Read the model definition and answer for the solid it produces. Units are mm, in the model's axes. Round coordinates to 2 decimals unless told otherwise and drop trailing zeros. Order: outer loops, then holes, each group sorted by start corner. A loop starts at its lowest first (then second) coordinate and runs counter-clockwise, first axis right, second up. Notation, with made-up numbers: (51.5, 25) - (92.5, 25) arc R28 ccw to (92.5, 45) - close; hole circle Ø9 at (86, 22.5). An arc over 180 degrees is marked (long way). Put each result on its own line as item: value. Start each with the question number.
Q1. Section B-B on y = -107.5 is taken. Give the vertices of the cut face in (x, z), then the cut area to 3 significant figures.
Q2. Section C-C on z = 100 is taken. Give the vertices of the cut face in (x, y), then the cut area to 3 significant figures.
Q3. Section A-A on z = -730.5 is taken. Give the vertices of the cut face in (x, y), then the cut area to 3 significant figures.
Q4. Each of these flat-tipped pins is pushed along its axis until it touches: pin 1 Ø5 at (x, y) = (422.5, -30.5) entering from +Z; pin 2 Ø3 at (y, z) = (-62, 583.5) entering from +X; pin 3 Ø1.5 at (x, y) = (-468, -133) entering from +Z. Where does it stop, or does it pass through?
Q5. Section D-D on x = 264 is taken. Give the vertices of the cut face in (y, z), then the cut area to 3 significant figures.
Q6. Find the intervals of material crossed by line 1 along X through (y, z) = (-67, -637); line 2 along Z through (x, y) = (-70.5, -88.5); line 3 along X through (y, z) = (-120.5, 274), in increasing order. Write a range as from..to.
from build123d import *

# Parameters (mm, degrees)
F1_DEPTH = 152.4
F2_W     = 1219.2
F2_H     = 1828.8
F3_DEPTH = 25.4
F4_DEPTH = 152.401


with BuildPart() as f1:
    # F0 (on Front) → F1 (new body)
    with BuildSketch(Plane.XZ):
        with BuildLine():
            Line((-962.472789, 62.231022), (-962.472789, -1309.368978))
            Line((-962.472789, -1309.368978), (866.327211, -1309.368978))
            Line((866.327211, -1309.368978), (866.327211, 62.231022))
            ThreePointArc((866.327211, 62.231022), (-48.072789, 976.631022), (-962.472789, 62.231022))
        make_face()
    extrude(amount=F1_DEPTH)

    # F2 (on face) → F3 (cut)
    with BuildSketch(Plane.XZ.offset(152.4)):
        with Locations((-48.072789, -394.968978)):
            Rectangle(F2_W, F2_H)
    extrude(amount=-F3_DEPTH, mode=Mode.SUBTRACT)

    # F2 (on face) → F4 (cut, through all)
    with BuildSketch(Plane.XZ.offset(152.4)):
        with Locations((-48.072789, -394.968978)):
            Rectangle(F2_W, F2_H)
    extrude(amount=-F4_DEPTH, mode=Mode.SUBTRACT)


solid = f1.part
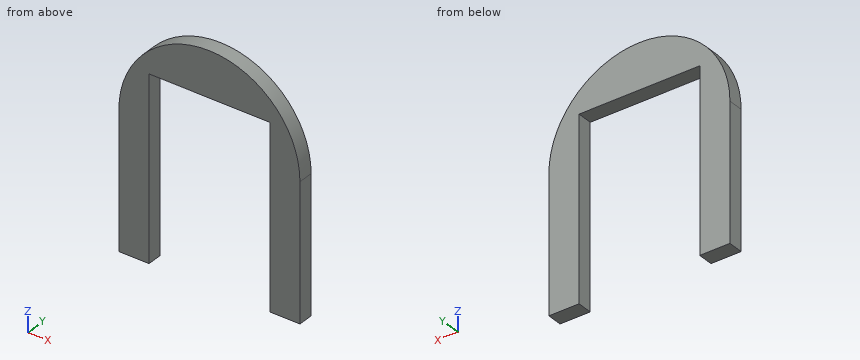
Findings:
1. outline: (-962.47, -1309.37) - (-657.67, -1309.37) - (-657.67, 519.43) - (561.53, 519.43) - (561.53, -1309.37) - (866.33, -1309.37) - (866.33, 62.23) arc R914.4 ccw to (-962.47, 62.23) - close
1. area: 1,590,000 mm2
2. outline: (-961.69, -152.4) - (-657.67, -152.4) - (-657.67, 0) - (-961.69, 0) - close; (561.53, -152.4) - (865.55, -152.4) - (865.55, 0) - (561.53, 0) - close
2. area: 92,700 mm2
3. outline: (-962.47, -152.4) - (-657.67, -152.4) - (-657.67, 0) - (-962.47, 0) - close; (561.53, -152.4) - (866.33, -152.4) - (866.33, 0) - (561.53, 0) - close
3. area: 92,900 mm2
4. pin 1: z = 847.75
4. pin 2: x = 704.24
4. pin 3: z = 874.89
5. outline: (-152.4, 519.43) - (0, 519.43) - (0, 921.73) - (-152.4, 921.73) - close
5. area: 61,300 mm2
6. line 1: -962.47..-657.67, 561.53..866.33
6. line 2: 519.43..976.36
6. line 3: -937.61..-657.67, 561.53..841.47
